For this review, take the finished solid that the model builds, in its own axes (mm). Coordinates: 2 decimals unless noted, no trailing zeros. Loops run counter-clockwise (first coordinate to the right, second up) from the corner with the lowest first, then second, coordinate; pieces in that order, holes last.
Autodesk Inventor part; units mm, degrees
ref_plane "YZ Plane" through (0, 0, 0) normal (1, 0, 0) x (0, 1, 0)
ref_plane "XZ Plane" through (0, 0, 0) normal (0, 1, 0) x (-1, 0, 0)
ref_plane "XY Plane" through (0, 0, 0) normal (0, 0, 1) x (1, 0, 0)
sketch "Sketch1" plane through (0, 0, 0) normal (1, 0, 0) x (0, 1, 0)
  circle A0 centre (0, 0) radius 75
  circle A1 centre (0, 0) radius 50
  dimension "d0" = 150
  dimension "d1" = 100
extrude "Extrusion1" add sketch "Sketch1" along normal blind 2
sketch "Sketch2" plane through (0, 0, 0) normal (-1, 0, 0) x (0, 0, 1)
  circle A0 centre (0, 0) radius 75
  line L0 (-75, 0) -> (-50, 0)
  circle A1 centre (0, 0) radius 50
  circle A2 centre (-62.5, 0) radius 4
  dimension "d4" = 8
extrude "Extrusion2" cut sketch "Sketch2" against normal blind 2 contours A2 L0 | L0 A2
pattern_circular "Circular Pattern1" count 6 over 360 about axis through (0, 0, 0) along (1, 0, 0) of "Extrusion2"
properties part number "11_Dem_cua_tham"
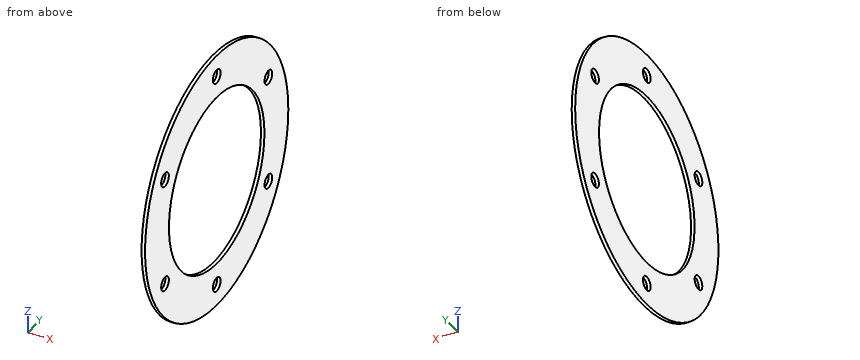
Q1. Consider section B-B (y = 53). State the section outline as (x, z) points, then the cut area to 3 significant figures.
Q2. For pin 1 Ø1 at (x, z) = (0.5, -38) entering from +Y, flat-tipped, find the tip position at first contact; note if it passes through.
Q3. Wall thickness on probe 1 along Z at (x, y) = (1.05, 0); probe 2 along Z at (x, y) = (0.9, 34); probe 3 along Z at (x, y) = (0.8, 12.5): over which ranges is each line inside the solid? List them lowest first.
Q4. Consider section A-A (z = 0). State the section outline as (x, y) points.
Q5. Consider section C-C (x = 0.3). State the section outline as (y, z) points.
Q6. Consider section D-D (y = -43.5). State the section outline as (x, z) points.
Model answer:
1. outline: (0, -53.07) - (2, -53.07) - (2, -35.09) - (0, -35.09) - close; (0, -27.41) - (2, -27.41) - (2, 27.41) - (0, 27.41) - close; (0, 35.09) - (2, 35.09) - (2, 53.07) - (0, 53.07) - close
1. area: 182 mm2
2. pin 1: stops at y = 64.95
3. probe 1: z = -75 to -66.5, -58.5 to -50, 50 to 58.5, 66.5 to 75
3. probe 2: z = -66.85 to -36.66, 36.66 to 66.85
3. probe 3: z = -73.95 to -48.41, 48.41 to 73.95
4. outline: (0, -75) - (2, -75) - (2, -50) - (0, -50) - close; (0, 50) - (2, 50) - (2, 75) - (0, 75) - close
5. outline: circle Ø150 at (0, 0); hole circle Ø8 at (-54.13, -31.25); hole circle Ø8 at (-54.13, 31.25); hole circle Ø100 at (0, 0); hole circle Ø8 at (0, -62.5); hole circle Ø8 at (0, 62.5); hole circle Ø8 at (54.13, -31.25); hole circle Ø8 at (54.13, 31.25)
6. outline: (0, -61.1) - (2, -61.1) - (2, -24.65) - (0, -24.65) - close; (0, 24.65) - (2, 24.65) - (2, 61.1) - (0, 61.1) - close
